```python
from build123d import *

# Parameters (mm, degrees)
SKETCH1_R           = 1.960784314
SKETCH1_W           = 23
SKETCH1_H           = 12
BOSS_EXTRUDE1_DEPTH = 5
FILLET2_R           = 20
SKETCH3_R           = 19.722379498
SKETCH3_R_2         = 3
BOSS_EXTRUDE2_DEPTH = 5
FILLET3_R           = 10
SKETCH6_R           = 4.5
CUT_EXTRUDE3_DEPTH  = 6
SKETCH7_R           = 1.5
SKETCH7_R_2         = 4.5
CUT_EXTRUDE4_DEPTH  = 10
SKETCH9_R           = 1.1
CUT_EXTRUDE6_DEPTH  = 10


with BuildPart() as part:
    # Sketch1 → Boss-Extrude1 (new body)
    with BuildSketch(Plane.XY):
        Polygon((49.019607843, 13.071895425), (49.019607843, -13.071895425), (-49.019607843, -9.803921569), (-50.980392157, -9.803921569), (-50.980392157, 9.803921569), (-49.019607843, 9.803921569), align=None)
        with Locations((43.790849673, 0)):
            Circle(SKETCH1_R, mode=Mode.SUBTRACT)
        with Locations((-32.679738562, 0)):
            Rectangle(SKETCH1_W, SKETCH1_H, mode=Mode.SUBTRACT)
    extrude(amount=BOSS_EXTRUDE1_DEPTH)

    # Fillet2
    # the kernel refuses this fillet: 20 mm, written as the material it takes off along each edge
    with BuildSketch(Plane(origin=(49.019607843, -13.071895425, -51.694436733), x_dir=(0, 1, 0), z_dir=(0, 0, 1))) as fillet2_piece_1:
        with BuildLine():
            CenterArc((FILLET2_R * 1.03388873465, FILLET2_R), FILLET2_R, 178.090847567, 91.909152433)
            Line((FILLET2_R * 0.0344438276744, FILLET2_R * 1.03331483023), (0, 0))
            Line((0, 0), (FILLET2_R * 1.03388873465, 0))
        make_face()
    extrude(amount=108.388873465, mode=Mode.SUBTRACT)
    with BuildSketch(Plane(origin=(49.019607843, 13.071895425, -51.694436733), x_dir=(0, -1, 0), z_dir=(0, 0, 1))) as fillet2_piece_2:
        with BuildLine():
            CenterArc((FILLET2_R * 1.03388873465, -FILLET2_R), FILLET2_R, 90, 91.909152433)
            Line((FILLET2_R * 0.0344438276744, -FILLET2_R * 1.03331483023), (0, 0))
            Line((0, 0), (FILLET2_R * 1.03388873465, 0))
        make_face()
    extrude(amount=108.388873465, mode=Mode.SUBTRACT)

    # Sketch3 → Boss-Extrude2 (add)
    with BuildSketch(Plane.XY.offset(5)):
        with Locations((43.790849673, 0)):
            Circle(SKETCH3_R)
        with Locations((43.790849673, 0)):
            Circle(SKETCH3_R_2, mode=Mode.SUBTRACT)
    extrude(amount=-BOSS_EXTRUDE2_DEPTH)

    # Fillet3
    fillet3_edges = [part.edges().sort_by_distance(p)[0] for p in [
        (-50.980392157, 9.803921569, 2.5),
        (-50.980392157, -9.803921569, 2.5),
        (28.442748303, -12.385799828, 2.5),
        (28.442748303, 12.385799828, 2.5),
    ]]
    fillet(fillet3_edges, radius=FILLET3_R)

    # Sketch6 → Cut-Extrude3 (cut)
    with BuildSketch(Plane.XY.offset(5)):
        with Locations((43.790849673, 0)):
            Circle(SKETCH6_R)
    extrude(amount=-CUT_EXTRUDE3_DEPTH, mode=Mode.SUBTRACT)

    # Sketch7 → Cut-Extrude4 (cut)
    with BuildSketch(Plane.XY.offset(5)):
        with Locations((53.608271623, 9.266511008)):
            Circle(SKETCH7_R)
        with Locations((43.790849673, 0)):
            Circle(SKETCH7_R_2)
        with Locations((56.724594586, -3.868881304)):
            Circle(SKETCH7_R)
        with Locations((46.907172636, -13.135392312)):
            Circle(SKETCH7_R)
        with Locations((33.973427724, -9.266511008)):
            Circle(SKETCH7_R)
        with Locations((30.857104761, 3.868881304)):
            Circle(SKETCH7_R)
        with Locations((40.67452671, 13.135392312)):
            Circle(SKETCH7_R)
    extrude(amount=-CUT_EXTRUDE4_DEPTH, mode=Mode.SUBTRACT)

    # Sketch9 → Cut-Extrude6 (cut)
    with BuildSketch(Plane.XY.offset(5)):
        with Locations((-46.829738562, 0)):
            Circle(SKETCH9_R)
        with Locations((-18.529738562, 0)):
            Circle(SKETCH9_R)
    extrude(amount=-CUT_EXTRUDE6_DEPTH, mode=Mode.SUBTRACT)


solid = part.part
```
For this review, take the finished solid that the model builds, in its own axes (mm). A direction names the side the tool comes from. Coordinates: 2 decimals unless noted, no trailing zeros. Loops run counter-clockwise (first coordinate to the right, second up) from the corner with the lowest first, then second, coordinate; pieces in that order, holes last. Notation, with made-up numbers: (7.5, 58) -> (54.5, 58) arc R17 ccw to (54.5, 65) -> close; hole circle Ø2 at (-39.75, -10.5). An arc over 180 degrees is marked (long way). Return JSON: item names as keys, results as strings. Group by question number.
(1) To check wall thickness, follow L1, parallel to X at y = 1, z = 3.9; L2, parallel to X at y = 4, z = 0.2; L3, parallel to Y at x = -41, z = 0.55. State the ranges of each line that lie inside material, in increasing order.
(2) Consider section A-A, the plane x = 40.5. Give the boundary of the cut face in (y, z), plus the area to 3 significant figures.
(3) Consider section B-B, the plane z = 1.3. Count the separate pieces of the cut face and the enclosed holes in it, plus the area to 3 significant figures.
(4) Tool access review of faces 1 (the flat face through (18, 0, 0)), 2 (the flat face through (-44.18, 0, 2)): name each direction out of +Z, -Z, +X, -X, +Y, -Y from which nothing blocks a thin tool from reaching the whole face with its end or side.
(5) Mouldability with a two-part tool opening along Y and no side actions: class faces 3 (the flat face through (18, 0, 5)), 4 (the cylindrical face through (63.503, -0.634, 2.535)), 5 (the cylindrical face through (32.8, -10.2, 2.5)) as pulls with the +Y half, pulls with the -Y half, needs draft (parallel to the pull), parting line crosses it, or undercut.
(6) For pin 1 Ø2 at (x, y) = (-46.83, 0) entering from -Z; pin 2 Ø2 at (x, z) = (-30, 2) entering from +Y; pin 3 Ø1.5 at (y, z) = (-11, 4) entering from +X; pin 4 Ø1.5 at (y, z) = (-12.5, 2.5) entering from +X, all flat-tipped, find the tip position at first contact; note any pin that passes through.
Results below:
{
 "1": {"L1": "x = -50.94 to -47.29, -46.37 to -44.18, -21.18 to -18.99, -18.07 to 39.4, 48.18 to 63.49", "L2": "x = -50.17 to -44.18, -21.18 to 29.36, 32.35 to 41.73, 45.85 to 63.1", "L3": "y = -10.07 to -6, 6 to 10.07"},
 "2": {"outline": "(-19.45, 0) -> (-3.07, 0) -> (-3.07, 5) -> (-19.45, 5) -> close; (3.07, 0) -> (11.65, 0) -> (11.65, 5) -> (3.07, 5) -> close; (14.63, 0) -> (19.45, 0) -> (19.45, 5) -> (14.63, 5) -> close", "area": "149 mm2"},
 "3": {"separate pieces": "1", "enclosed holes": "10", "area": "2,480 mm2"},
 "4": {"face 1": "-Z, +X, -X, +Y, -Y", "face 2": "+Z, -Z"},
 "5": {"face 3": "needs draft", "face 4": "parting line crosses it", "face 5": "undercut"},
 "6": {"pin 1": "passes through", "pin 2": "stops at y = 10.47", "pin 3": "stops at x = 60.64", "pin 4": "stops at x = 59.63"}
}
